Source: CAD feature listing. Evaluate the final solid. Frame: model axes, mm. A direction names the side the tool comes from. Coordinates: 2 decimals unless noted, no trailing zeros. Loops run counter-clockwise (first coordinate to the right, second up) from the corner with the lowest first, then second, coordinate; pieces in that order, holes last.
from build123d import *

# Parameters (mm, degrees)
SKETCH1_R           = 1.737885662
SKETCH1_R_2         = 1.873200063
SKETCH1_R_3         = 1.690089146
SKETCH1_R_4         = 1.754205974
SKETCH1_R_5         = 1.7
SKETCH1_R_6         = 4.5
SKETCH1_R_7         = 1.87
SKETCH1_R_8         = 9.5
SKETCH1_W           = 3
SKETCH1_H           = 10
SKETCH1_W_2         = 10
SKETCH1_H_2         = 3
BOSS_EXTRUDE1_DEPTH = 3
FILLET1_R           = 3
FILLET2_R           = 10


with BuildPart() as part:
    # Sketch1 → Boss-Extrude1 (new body)
    with BuildSketch(Plane.XY):
        Polygon((147.061964125, -92.970138098), (147.061964125, -71.856515964), (147.061964125, -67.856515964), (175.843347401, -67.856515964), (175.843347401, -87.856515964), (183.843347401, -87.856515964), (183.843347401, -135.887076434), (175.843347401, -135.887076434), (175.843347401, -155.887076434), (147.061964125, -155.887076434), (147.061964125, -151.887076434), (147.061964125, -130.215533927), (127.203791419, -130.215533927), (127.203791419, -111.591712302), (127.203791419, -92.970138098), align=None)
        with Locations((130.520049527, -96.082032258)):
            Circle(SKETCH1_R, mode=Mode.SUBTRACT)
        with Locations((161.520049527, -96.082032258)):
            Circle(SKETCH1_R_2, mode=Mode.SUBTRACT)
        with Locations((130.520049527, -127.114221831)):
            Circle(SKETCH1_R_3, mode=Mode.SUBTRACT)
        with Locations((161.520049527, -127.082032258)):
            Circle(SKETCH1_R_4, mode=Mode.SUBTRACT)
        with Locations((154.157584865, -111.662272701)):
            Circle(SKETCH1_R_5, mode=Mode.SUBTRACT)
        with Locations((145.89014032, -119.788596448)):
            Circle(SKETCH1_R_5, mode=Mode.SUBTRACT)
        with Locations((137.763816574, -111.521151903)):
            Circle(SKETCH1_R_5, mode=Mode.SUBTRACT)
        with Locations((146.031261118, -103.394828157)):
            Circle(SKETCH1_R_5, mode=Mode.SUBTRACT)
        with Locations((145.960700719, -111.591712302)):
            Circle(SKETCH1_R_6, mode=Mode.SUBTRACT)
        with Locations((175.843347401, -96.114221831)):
            Circle(SKETCH1_R_7, mode=Mode.SUBTRACT)
        with Locations((157.960700719, -81.591712302)):
            Circle(SKETCH1_R_8, mode=Mode.SUBTRACT)
        with Locations((157.960700719, -141.591712302)):
            Circle(SKETCH1_R_8, mode=Mode.SUBTRACT)
        with Locations((175.843347401, -127.114221831)):
            Circle(SKETCH1_R_7, mode=Mode.SUBTRACT)
        with Locations((131.960700719, -111.591712302)):
            Rectangle(SKETCH1_W, SKETCH1_H, mode=Mode.SUBTRACT)
        with Locations((145.960700719, -97.591712302)):
            Rectangle(SKETCH1_W_2, SKETCH1_H_2, mode=Mode.SUBTRACT)
        with Locations((145.960700719, -125.591712302)):
            Rectangle(SKETCH1_W_2, SKETCH1_H_2, mode=Mode.SUBTRACT)
        with Locations((166.293610901, -111.591712302)):
            Rectangle(SKETCH1_W, SKETCH1_H, mode=Mode.SUBTRACT)
    extrude(amount=BOSS_EXTRUDE1_DEPTH)

    # Fillet1
    fillet1_edges = [part.edges().sort_by_distance(p)[0] for p in [
        (175.843347401, -87.856515964, 1.5),
        (183.843347401, -87.856515964, 1.5),
        (183.843347401, -135.887076434, 1.5),
        (175.843347401, -135.887076434, 1.5),
        (147.061964125, -130.215533927, 1.5),
        (127.203791419, -130.215533927, 1.5),
        (127.203791419, -92.970138098, 1.5),
        (147.061964125, -92.970138098, 1.5),
    ]]
    fillet(fillet1_edges, radius=FILLET1_R)

    # Fillet2
    fillet2_edges = [part.edges().sort_by_distance(p)[0] for p in [
        (147.061964125, -67.856515964, 1.5),
        (175.843347401, -67.856515964, 1.5),
        (175.843347401, -155.887076434, 1.5),
        (147.061964125, -155.887076434, 1.5),
    ]]
    fillet(fillet2_edges, radius=FILLET2_R)


solid = part.part
Q1. Draft query along X for faces 1 (the flat face through (147.062, -84, 1)), 2 (the flat face through (137, -92.97, 1)), 3 (the flat face through (130.461, -112, 1)), 4 (the cylindrical face through (148.38, -107.797, 1.479)). Return one class per face: +X half, -X half, draft (parallel to the pull), parting line (faces both ways), or undercut.
Q2. Line query: line 1 along Y through (x, z) = (158.5, 0.65); line 2 along X through (y, z) = (-125, 1.9); line 3 along Y through (x, z) = (166, 2.85). Output: solid intervals per line, ascending.
Q3. Contact query for flat-ended pins moving along their axis: pin 1 Ø0.9 at (x, z) = (136, 2) entering from -Y; pin 2 Ø1 at (y, z) = (-136.5, 1.5) entering from -X; pin 3 Ø3 at (x, y) = (137.76, -111.52) entering from -Z; pin 4 Ø0.9 at (x, z) = (144, 2) entering from +Y. Output: stop coordinate, or through.
Q4. Access query for faces 5 (the flat face through (162, -155.887, 1)), 6 (the cylindrical face through (182.99, -134.98, 1.52)), 7 (the flat face through (147.062, -139, 1)), 8 (the flat face through (166, -106.592, 1)), 9 (the flat face through (175.843, -81, 1)). Directions: +Z, -Z, +X, -X, +Y, -Y. A direction counts if a zero-diameter tool reaches every point of the face in a straight line with its end or side. Return the directions, or none.
Q5. Section D-D, the plane z = 2.05. Count the separate pieces of the cut face and the enclosed holes in it, plus the area to 3 significant figures.
Q6. Section A-A, the plane x = 142.5. Return the cut outline in (y, z), plus the area to 3 significant figures.
Q7. Section B-B, the plane y = -75.5. Return the cut outline in (x, z), plus the area to 3 significant figures.
Q8. Section C-C, the plane y = -140.5. Return the cut outline in (x, z), plus the area to 3 significant figures.
Derived:
1. face 1: -X half
1. face 2: draft
1. face 3: undercut
1. face 4: undercut
2. line 1: y = -155.89 to -151.08, -132.11 to -91.08, -72.11 to -67.86
2. line 2: x = 127.2 to 140.96, 150.96 to 183.84
2. line 3: y = -155.89 to -146.65, -136.53 to -116.59, -106.59 to -86.65, -76.53 to -67.86
3. pin 1: stops at y = -130.22
3. pin 2: stops at x = 147.06
3. pin 3: passes through
3. pin 4: stops at y = -92.94
4. face 5: +Z, -Z, +X, -X, -Y
4. face 6: +Z, -Z, +X, -Y
4. face 7: +Z, -Z, -X, -Y
4. face 8: +Z, -Z
4. face 9: +Z, -Z, +X, +Y
5. separate pieces: 1
5. enclosed holes: 17
5. area: 2,720 mm2
6. outline: (-130.22, 0) - (-127.09, 0) - (-127.09, 3) - (-130.22, 3) - close; (-124.09, 0) - (-114.47, 0) - (-114.47, 3) - (-124.09, 3) - close; (-108.72, 0) - (-99.09, 0) - (-99.09, 3) - (-108.72, 3) - close; (-96.09, 0) - (-92.97, 0) - (-92.97, 3) - (-96.09, 3) - close
6. area: 76.5 mm2
7. outline: (147.34, 0) - (150.67, 0) - (150.67, 3) - (147.34, 3) - close; (165.25, 0) - (175.56, 0) - (175.56, 3) - (165.25, 3) - close
7. area: 40.9 mm2
8. outline: (147.06, 0) - (148.52, 0) - (148.52, 3) - (147.06, 3) - close; (167.4, 0) - (175.84, 0) - (175.84, 3) - (167.4, 3) - close
8. area: 29.7 mm2
